CAD build for the part. Positions are in the model's coordinates, mm. Coordinates: 2 decimals unless noted, no trailing zeros. Order: outer loops, then holes, each group sorted by start corner. A loop starts at its lowest first (then second) coordinate and runs counter-clockwise, first axis right, second up. Notation, with made-up numbers: (35.5, 38.5) - (56.5, 38.5) arc R27 cw to (56.5, 63.5) - close; hole circle Ø1 at (85.25, 48.5). An arc over 180 degrees is marked (long way). Use one line per item in the form item = value.
```python
from build123d import *

# Parameters (mm, degrees)
F0_R     = 51.147265
F0_R_2   = 2.800835
F0_R_3   = 3
F0_R_4   = 18.413015
F1_DEPTH = 3


with BuildPart() as f1:
    # F0 (on Front) → F1 (new body)
    with BuildSketch(Plane.XZ):
        with Locations((-39.088421, 7.339887)):
            Circle(F0_R)
        with Locations((-60.588101, -29.89939)):
            Circle(F0_R_2, mode=Mode.SUBTRACT)
        with Locations((-60.588101, 44.579164)):
            Circle(F0_R_3, mode=Mode.SUBTRACT)
        with Locations((-39.088421, 7.339887)):
            Circle(F0_R_4, mode=Mode.SUBTRACT)
        with Locations((3.911579, 7.339887)):
            Circle(F0_R_2, mode=Mode.SUBTRACT)
    extrude(amount=F1_DEPTH)


solid = f1.part
```
Item 1: Drop flat-ended pins along their axis: pin 1 (1 mm diameter, centred on y = -2.5, z = -32, fed in from +X); pin 2 (1.5 mm diameter, centred on x = -26, y = -2, fed in from -Z); pin 3 (1.5 mm diameter, centred on y = -2, z = 18.5, fed in from +X). Give the stop position or say it passes through.
Derived:
pin_1 = -5.81
pin_2 = -42.3
pin_3 = 10.99
Item 2: Drill centre lines: line 1 (X direction, y = -2.3, z = 5); line 2 (X direction, y = -2.65, z = 20); line 3 (X direction, y = -2.4, z = 15). Where is each one in solid material? Low to high. Write a range as [from, to].
Derived:
line_1 = [-90.18, -57.35], [-20.82, 2.37], [5.45, 12.01]
line_2 = [-88.64, -52.46], [-25.72, 10.47]
line_3 = [-89.66, -55.83], [-22.34, 11.48]
Item 3: Two-plate mould, pull along Z, no slides. Class faces 1 (the face through (1.113, -1.479, 7.463)), 2 (the face through (8.16, -1.48, -12.25)), 3 (the face through (-40, -3, -15)): +Z half, -Z half, draft (parallel to the pull), parting line (faces both ways), or undercut.
Derived:
face_1 = undercut
face_2 = parting line
face_3 = draft
Item 4: Cut at D-D, the plane y = -1.2. Write the cut outline in (x, z), plus the area to 3 significant figures.
Derived:
outline = circle Ø102.29 at (-39.09, 7.34); hole circle Ø6 at (-60.59, 44.58); hole circle Ø5.6 at (-60.59, -29.9); hole circle Ø36.83 at (-39.09, 7.34); hole circle Ø5.6 at (3.91, 7.34)
area = 7,080 mm²
Item 5: Cut at B-B, the plane z = 3. Write the cut outline in (x, y).
Derived:
outline = (-90.05, -3) - (-56.98, -3) - (-56.98, 0) - (-90.05, 0) - close; (-21.19, -3) - (11.87, -3) - (11.87, 0) - (-21.19, 0) - close
Item 6: Cut at C-C, the plane x = -46. Write the cut outline in (y, z), plus the area to 3 significant figures.
Derived:
outline = (-3, -43.34) - (0, -43.34) - (0, -9.73) - (-3, -9.73) - close; (-3, 24.41) - (0, 24.41) - (0, 58.02) - (-3, 58.02) - close
area = 202 mm²
Item 7: Cut at A-A, the plane x = -60.5. Write the cut outline in (y, z).
Derived:
outline = (-3, -39.11) - (0, -39.11) - (0, -32.7) - (-3, -32.7) - close; (-3, -27.1) - (0, -27.1) - (0, 41.58) - (-3, 41.58) - close; (-3, 47.58) - (0, 47.58) - (0, 53.79) - (-3, 53.79) - close
